from build123d import *

# Parameters (mm, degrees)
SKETCH1_R           = 4.7625
SKETCH1_R_2         = 3.175
BOSS_EXTRUDE1_DEPTH = 25.4
SKETCH1_3_R         = 4.7625
CUT_EXTRUDE1_DEPTH  = 16.51
SKETCH2_R           = 3.175
CUT_EXTRUDE2_DEPTH  = 17.78
SKETCH3_W           = 25.4
SKETCH3_H           = 9.525
CUT_EXTRUDE3_DEPTH  = 6.35


with BuildPart() as part:
    # Sketch1 → Boss-Extrude1 (new body)
    with BuildSketch(Plane.XY):
        with BuildLine():
            ThreePointArc((-12.7, 99.06), (-9.724204897, 106.244204897), (-2.54, 109.22))
            Line((-2.54, 109.22), (2.54, 109.22))
            ThreePointArc((2.54, 109.22), (9.724204897, 106.244204897), (12.7, 99.06))
            Line((12.7, 99.06), (12.7, 0))
            Line((12.7, 0), (-12.7, 0))
            Line((-12.7, 0), (-12.7, 99.06))
        make_face()
        with Locations((0, 101.346)):
            Circle(SKETCH1_R, mode=Mode.SUBTRACT)
        with Locations((6.35, 86.36)):
            Circle(SKETCH1_R_2, mode=Mode.SUBTRACT)
        with Locations((-6.35, 86.36)):
            Circle(SKETCH1_R_2, mode=Mode.SUBTRACT)
        with Locations((0, 32.385)):
            Circle(SKETCH1_R, mode=Mode.SUBTRACT)
        with Locations((0, 101.346)):
            Circle(SKETCH1_R)
    extrude(amount=-BOSS_EXTRUDE1_DEPTH)

    # Sketch1_3 → Cut-Extrude1 (cut)
    with BuildSketch(Plane.XY):
        with Locations((0, 101.346)):
            Circle(SKETCH1_3_R)
    extrude(amount=-CUT_EXTRUDE1_DEPTH, mode=Mode.SUBTRACT)

    # Sketch2 → Cut-Extrude2 (cut)
    with BuildSketch(Plane.XZ):
        with Locations((0, -12.7)):
            Circle(SKETCH2_R)
    extrude(amount=-CUT_EXTRUDE2_DEPTH, mode=Mode.SUBTRACT)

    # Sketch3 → Cut-Extrude3 (cut)
    with BuildSketch(Plane.XY):
        with Locations((0, 46.0375)):
            Rectangle(SKETCH3_W, SKETCH3_H)
        with Locations((0, 18.7325)):
            Rectangle(SKETCH3_W, SKETCH3_H)
    extrude(amount=-CUT_EXTRUDE3_DEPTH, mode=Mode.SUBTRACT)


solid = part.part
For this review, take the finished solid that the model builds, in its own axes (mm). A direction names the side the tool comes from. Give positions to 0.01 mm unless a question says otherwise; leave off trailing zeros. Order: outer loops, then holes, each group sorted by start corner. A loop starts at its lowest first (then second) coordinate and runs counter-clockwise, first axis right, second up. Notation, with made-up numbers: (46.25, 88) - (58.25, 88) arc R21 ccw to (58.25, 99) - close; hole circle Ø9 at (-32.5, 77.5). An arc over 180 degrees is marked (long way). Answer as a JSON object with one key per item and string values. Group by question number.
Item 1: Take a section at B-B on x = -6.35. Give the boundary of the cut face in (y, z) (3 decimals), and give its area (3 significant figures).
Item 2: Wall thickness on line 1 along Y through (x, z) = (0, -13.25); line 2 along Y through (x, z) = (0, -16); line 3 along Z through (x, y) = (0, 5.75) (3 decimals): over which ranges is each line inside the solid? List them lowest first.
Item 3: Take a section at A-A on y = 86.36. Give the boundary of the cut face in (x, z) (3 decimals).
Item 4: Clearance check with flat-ended pins moving along their axes: pin 1 Ø6 at (x, y) = (-3.5, 75) entering from +Z; pin 2 Ø1 at (x, z) = (-6.5, -18.5) entering from +Y; pin 3 Ø4 at (x, y) = (-6.35, 86.36) entering from +Z; pin 4 Ø3 at (x, y) = (1.5, 45) entering from +Z. State where each tip first meets the part, or that it passes through.
Item 5: Draft analysis for pull direction X (two halves, no side actions). For faces 6 (the flat face through (0, 41.275, -3)), 7 (the flat face through (0, 101, -16.51)), 8 (the flat face through (-12.7, 49, -13)), state which applies: pulls with the +X half, pulls with the -X half, needs draft (parallel to the pull), parting line crosses it, or undercut.
Item 6: Take a section at C-C on z = -2.25. Give the number of separate pieces and of enclosed holes in the cut face, and give its area (3 significant figures).
Item 7: Machinability: for faces 1 (the cylindrical face through (-0.69, 8.77, -15.8)), 2 (the cylindrical face through (5.66, 83.26, -12.52)), 3 (the flat face through (0, 46, -6.35)), 4 (the flat face through (0, 109.22, -13)), 5 (the cylindrical face through (-0.62, 106.068, -8.139)), which of the approach directions +Z, -Z, +X, -X, +Y, -Y give a long, thin tool a straight path to every point of the face, cutting with its end or side? Answer none if there is none.
Reported:
{
 "1": {"outline": "(0, -25.4) - (83.185, -25.4) - (83.185, 0) - (50.8, 0) - (50.8, -6.35) - (41.275, -6.35) - (41.275, 0) - (23.495, 0) - (23.495, -6.35) - (13.97, -6.35) - (13.97, 0) - (0, 0) - close; (89.535, -25.4) - (108.479, -25.4) - (108.479, 0) - (89.535, 0) - close", "area": "2,470 mm^2"},
 "2": {"line 1": "17.78 to 27.62, 37.15 to 96.58, 106.11 to 109.22", "line 2": "0 to 27.62, 37.15 to 96.58, 106.11 to 109.22", "line 3": "-25.4 to -15.875, -9.525 to 0"},
 "3": {"outline": "(-12.7, -25.4) - (-9.525, -25.4) - (-9.525, 0) - (-12.7, 0) - close; (-3.175, -25.4) - (3.175, -25.4) - (3.175, 0) - (-3.175, 0) - close; (9.525, -25.4) - (12.7, -25.4) - (12.7, 0) - (9.525, 0) - close"},
 "4": {"pin 1": "z = 0", "pin 2": "y = 108.61", "pin 3": "through", "pin 4": "z = -6.35"},
 "5": {"face 6": "needs draft", "face 7": "undercut", "face 8": "pulls with the -X half"},
 "6": {"separate pieces": "3", "enclosed holes": "4", "area": "2,040 mm^2"},
 "7": {"face 1": "-Y", "face 2": "+Z, -Z", "face 3": "+Z, +X, -X", "face 4": "+Z, -Z, +X, -X, +Y", "face 5": "+Z"}
}
